```python
from build123d import *

# Parameters (mm, degrees)
BOX237_W           = 6
BOX237_H           = 6
BOX237_DEPTH       = 64
BOX236_W           = 6
BOX236_H           = 6
BOX236_DEPTH       = 64
CYLINDER1243_R     = 3
CYLINDER1243_DEPTH = 3
CYLINDER1242_R     = 3
CYLINDER1242_DEPTH = 3
CYLINDER1257_R     = 1.5
CYLINDER1257_DEPTH = 32
CYLINDER1256_R     = 1.5
CYLINDER1256_DEPTH = 32
CYLINDER1255_R     = 1.5
CYLINDER1255_DEPTH = 100
CYLINDER1254_R     = 1.5
CYLINDER1254_DEPTH = 100
CYLINDER1248_R     = 1.5
CYLINDER1248_DEPTH = 50
CYLINDER1250_R     = 1.5
CYLINDER1250_DEPTH = 50
CYLINDER1251_R     = 1.5
CYLINDER1251_DEPTH = 50
CYLINDER1249_R     = 1.5
CYLINDER1249_DEPTH = 50
CYLINDER1246_R     = 1.5
CYLINDER1246_DEPTH = 100
CYLINDER1247_R     = 1.5
CYLINDER1247_DEPTH = 100
CYLINDER1252_R     = 1.5
CYLINDER1252_DEPTH = 100
CYLINDER1253_R     = 1.5
CYLINDER1253_DEPTH = 100
BOX139_W           = 200
BOX139_H           = 100
BOX139_DEPTH       = 32
TUBE001_R          = 59
TUBE001_R_2        = 40
TUBE001_DEPTH      = 10


with BuildPart() as krychle237:
    # Box237 → Box237 (new body)
    with BuildSketch(Plane(origin=(87, -3, -93), x_dir=(1, 0, 0), z_dir=(0, 0, 1))):
        with Locations((3, 3)):
            Rectangle(BOX237_W, BOX237_H)
    extrude(amount=BOX237_DEPTH)


with BuildPart() as compound627:
    # Box236 → Box236 (new body)
    with BuildSketch(Plane(origin=(11, -3, -93), x_dir=(1, 0, 0), z_dir=(0, 0, 1))):
        with Locations((3, 3)):
            Rectangle(BOX236_W, BOX236_H)
    extrude(amount=BOX236_DEPTH)

    # Compound627: union Krychle237
    add(krychle237.part)


with BuildPart() as compound627_1:
    # Compound627 placement: moved
    add(compound627.part.moved(Location((-52, 0, 36))))


with BuildPart() as obj1:
    # Cylinder1243 → Cylinder1243 (new body)
    with BuildSketch(Plane(origin=(78, 41, -42), x_dir=(1, 0, 0), z_dir=(0, 0, 1))):
        Circle(CYLINDER1243_R)
    extrude(amount=CYLINDER1243_DEPTH)


with BuildPart() as compound633:
    # Cylinder1242 → Cylinder1242 (new body)
    with BuildSketch(Plane(origin=(26, 41, -42), x_dir=(1, 0, 0), z_dir=(0, 0, 1))):
        Circle(CYLINDER1242_R)
    extrude(amount=CYLINDER1242_DEPTH)

    # Compound633: union obj1
    add(obj1.part)


with BuildPart() as compound633_1:
    # Compound633 placement: moved
    add(compound633.part.moved(Location((-52, 0, 42))))


with BuildPart() as obj2:
    # Cylinder1257 → Cylinder1257 (new body)
    with BuildSketch(Plane(origin=(78, 41, -42), x_dir=(1, 0, 0), z_dir=(0, 0, 1))):
        Circle(CYLINDER1257_R)
    extrude(amount=CYLINDER1257_DEPTH)


with BuildPart() as compound641:
    # Cylinder1256 → Cylinder1256 (new body)
    with BuildSketch(Plane(origin=(26, 41, -42), x_dir=(1, 0, 0), z_dir=(0, 0, 1))):
        Circle(CYLINDER1256_R)
    extrude(amount=CYLINDER1256_DEPTH)

    # Compound641: union obj2
    add(obj2.part)


with BuildPart() as compound641_1:
    # Compound641 placement: moved
    add(compound641.part.moved(Location((-52, 0, 36))))


with BuildPart() as obj3:
    # Cylinder1255 → Cylinder1255 (new body)
    with BuildSketch(Plane(origin=(14, 0, -60), x_dir=(1, 0, 0), z_dir=(0, 0, 1))):
        Circle(CYLINDER1255_R)
    extrude(amount=CYLINDER1255_DEPTH)


with BuildPart() as compound639:
    # Cylinder1254 → Cylinder1254 (new body)
    with BuildSketch(Plane(origin=(90, 0, -60), x_dir=(1, 0, 0), z_dir=(0, 0, 1))):
        Circle(CYLINDER1254_R)
    extrude(amount=CYLINDER1254_DEPTH)

    # Compound640: union obj3
    add(obj3.part)


with BuildPart() as compound639_1:
    # Compound640 placement: moved
    add(compound639.part.moved(Location((-52, 0, 0))))

    # Compound639: union Compound641
    add(compound641_1.part)


with BuildPart() as obj4:
    # Cylinder1248 → Cylinder1248 (new body)
    with BuildSketch(Plane(origin=(-51, 6, 0), x_dir=(1, 0, 0), z_dir=(0, 0, 1))):
        Circle(CYLINDER1248_R)
    extrude(amount=CYLINDER1248_DEPTH)


with BuildPart() as obj5:
    # Cylinder1250 → Cylinder1250 (new body)
    with BuildSketch(Plane(origin=(-24, 18, 0), x_dir=(1, 0, 0), z_dir=(0, 0, 1))):
        Circle(CYLINDER1250_R)
    extrude(amount=CYLINDER1250_DEPTH)


with BuildPart() as obj6:
    # Cylinder1251 → Cylinder1251 (new body)
    with BuildSketch(Plane(origin=(24, 18, 0), x_dir=(1, 0, 0), z_dir=(0, 0, 1))):
        Circle(CYLINDER1251_R)
    extrude(amount=CYLINDER1251_DEPTH)


with BuildPart() as compound637:
    # Cylinder1249 → Cylinder1249 (new body)
    with BuildSketch(Plane(origin=(51, 6, 0), x_dir=(1, 0, 0), z_dir=(0, 0, 1))):
        Circle(CYLINDER1249_R)
    extrude(amount=CYLINDER1249_DEPTH)

    # Compound637: union obj4, obj5, obj6
    add(obj4.part)
    add(obj5.part)
    add(obj6.part)


with BuildPart() as obj7:
    # Cylinder1246 → Cylinder1246 (new body)
    with BuildSketch(Plane(origin=(51, -12, 0), x_dir=(1, 0, 0), z_dir=(0, 0, 1))):
        Circle(CYLINDER1246_R)
    extrude(amount=CYLINDER1246_DEPTH)


with BuildPart() as compound636:
    # Cylinder1247 → Cylinder1247 (new body)
    with BuildSketch(Plane(origin=(-51, -12, 0), x_dir=(1, 0, 0), z_dir=(0, 0, 1))):
        Circle(CYLINDER1247_R)
    extrude(amount=CYLINDER1247_DEPTH)

    # Compound636: union obj7
    add(obj7.part)


with BuildPart() as obj8:
    # Cylinder1252 → Cylinder1252 (new body)
    with BuildSketch(Plane(origin=(39, -21, 0), x_dir=(1, 0, 0), z_dir=(0, 0, 1))):
        Circle(CYLINDER1252_R)
    extrude(amount=CYLINDER1252_DEPTH)


with BuildPart() as compound635:
    # Cylinder1253 → Cylinder1253 (new body)
    with BuildSketch(Plane(origin=(-39, -21, 0), x_dir=(1, 0, 0), z_dir=(0, 0, 1))):
        Circle(CYLINDER1253_R)
    extrude(amount=CYLINDER1253_DEPTH)

    # Compound638: union obj8
    add(obj8.part)

    # Compound635: union Compound637, Compound636
    add(compound637.part)
    add(compound636.part)


with BuildPart() as compound635_1:
    # Compound635 placement: moved
    add(compound635.part.moved(Location((0, 0, -10))))


with BuildPart() as krychle139:
    # Box139 → Box139 (new body)
    with BuildSketch(Plane(origin=(-100, -124, 0), x_dir=(1, 0, 0), z_dir=(0, 0, 1))):
        with Locations((100, 50)):
            Rectangle(BOX139_W, BOX139_H)
    extrude(amount=BOX139_DEPTH)


with BuildPart() as cut198:
    # Tube001 → Tube001 (new body)
    with BuildSketch(Plane.XY):
        Circle(TUBE001_R)
        Circle(TUBE001_R_2, mode=Mode.SUBTRACT)
    extrude(amount=TUBE001_DEPTH)

    # Cut191: cut Krychle139
    add(krychle139.part, mode=Mode.SUBTRACT)

    # Cut194: cut Compound635
    add(compound635_1.part, mode=Mode.SUBTRACT)

    # Cut195: cut Compound639
    add(compound639_1.part, mode=Mode.SUBTRACT)

    # Cut196: cut Compound633
    add(compound633_1.part, mode=Mode.SUBTRACT)

    # Cut198: cut Compound627
    add(compound627_1.part, mode=Mode.SUBTRACT)


solid = cut198.part
```
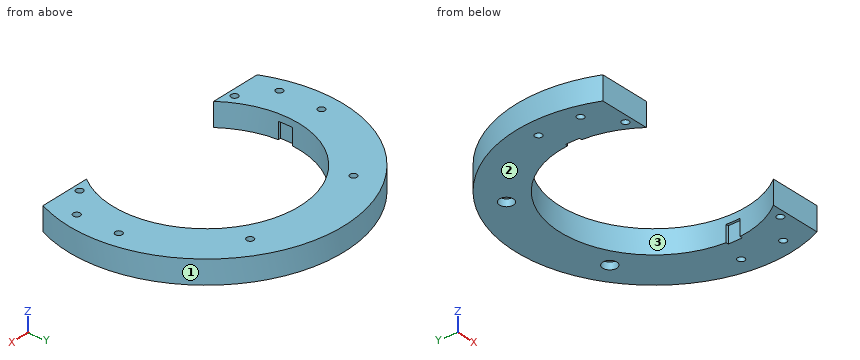
Design review of the part built by this model. Coordinates are the model's own, in mm. Face numbers are marked on the shaded views. Coordinates: 2 decimals unless noted, no trailing zeros. Write each loop counter-clockwise with the first axis right and the second up, starting at its lowest first coordinate (ties: lowest second). Pieces come first, ordered by that corner, then holes. Notation, with made-up numbers: M 76.5,48 L 91.5,48 A12 ccw 91.5,68 Z; hole C 21.25,56 d6. An arc over 180 degrees is marked long. Answer as a JSON object with one key per item and string values.
Item 1: Insertion check: pin 1 Ø3.5 at (x, y) = (-26, 41) entering from -Z; pin 2 Ø3 at (y, z) = (14, 6) entering from -X; pin 3 Ø0.9 at (x, y) = (40.5, -0.5) entering from -Z. Each pin has a flat end and moves straight along its axis. Give the tip position at first contact, or say it passes through.
Outcome:
{"pin 1": "z = 3", "pin 2": "x = -57.66", "pin 3": "z = 7"}
Item 2: Add section B-B, the plane x = 51. Give the boundary of the cut face in (y, z).
Outcome:
{"outline": "M -24,0 L -13.5,0 L -13.5,10 L -24,10 Z; M -10.5,0 L 4.5,0 L 4.5,10 L -10.5,10 Z; M 7.5,0 L 29.66,0 L 29.66,10 L 7.5,10 Z"}
Item 3: Wall thickness on probe 1 along X at (y, z) = (41, 7.5); probe 2 along X at (y, z) = (-21, 7.5); probe 3 along Y at (x, z) = (-50, 3.5): over which ranges is each line inside the solid? List them lowest first.
Outcome:
{"probe 1": "-42.43 to -27.5, -24.5 to 24.5, 27.5 to 42.43", "probe 2": "-55.14 to -40.5, -37.5 to -34.04, 34.04 to 37.5, 40.5 to 55.14", "probe 3": "-24 to -13.12, -10.88 to 4.88, 7.12 to 31.32"}
Item 4: Add section A-A, the plane y = 0. Give the boundary of the cut face in (x, z).
Outcome:
{"outline": "M -59,0 L -41,0 L -41,7 L -40,7 L -40,10 L -59,10 Z; M 40,7 L 41,7 L 41,0 L 59,0 L 59,10 L 40,10 Z"}
Item 5: Draft analysis for pull direction Y (two halves, no side actions). For the marked faces 1, 2 and 3, state which applies: pulls with the +Y half, pulls with the -Y half, needs draft (parallel to the pull), parting line crosses it, or undercut.
Outcome:
{"face 1": "parting line crosses it", "face 2": "needs draft", "face 3": "undercut"}
Item 6: Add section D-D, the plane y = -12. Give the boundary of the cut face in (x, z).
Outcome:
{"outline": "M -57.77,0 L -52.5,0 L -52.5,10 L -57.77,10 Z; M -49.5,0 L -38.16,0 L -38.16,10 L -49.5,10 Z; M 38.16,0 L 49.5,0 L 49.5,10 L 38.16,10 Z; M 52.5,0 L 57.77,0 L 57.77,10 L 52.5,10 Z"}
Item 7: Add section C-C, the plane x = -26. Give the boundary of the cut face in (y, z), and give its area (3 significant figures).
Outcome:
{"outline": "M 30.4,0 L 38,0 L 38,3 L 39.5,3 L 39.5,10 L 30.4,10 Z; M 42.5,3 L 44,3 L 44,0 L 52.96,0 L 52.96,10 L 42.5,10 Z", "area": "187 mm²"}
